Read the model definition and answer for the solid it produces. Units are mm, in the model's axes. A direction names the side the tool comes from. Coordinates: 2 decimals unless noted, no trailing zeros. Write each loop counter-clockwise with the first axis right and the second up, starting at its lowest first coordinate (ties: lowest second). Pieces come first, ordered by that corner, then holes.
(1) Find the intervals of material crossed by probe 1 along Y at (x, z) = (20, 2.4); probe 2 along Y at (x, z) = (0, 3.1); probe 3 along Y at (x, z) = (37, 3.55), in increasing order.
(2) Section D-D on x = 49 is taken. Write down the section's boundary in (y, z), then the cut area to 3 significant figures.
(3) The mould has two halves that part along Y. Classify faces 3 (the cylindrical face through (25.5, 0.07, 2.96)), 4 (the flat face through (30, 0, 6)), 5 (the flat face through (36, -6, 3)): +Y half, -Y half, draft (parallel to the pull), parting line (faces both ways), or undercut.
(4) Given pin 1 (2.5 mm diameter, centred on x = 60, y = 0, fed in from +Z); pin 2 (1.8 mm diameter, centred on x = 24.5, z = 3, fed in from -Y); pin 3 (1.5 mm diameter, centred on y = -2, z = 2, fed in from +X); pin 4 (1 mm diameter, centred on x = 9.5, z = 1, fed in from -Y), each flat-ended and moving along its own axis, determine where each tip first touches the part or whether it passes through.
(5) Section A-A on y = 0 is taken. Write down the section's boundary in (x, z).
(6) Section B-B on x = 20 is taken. Write down the section's boundary in (y, z), then the cut area to 3 significant figures.
(7) Which of the six approach directions +Z, -Z, +X, -X, +Y, -Y give full straight-line access (tool end or side, diameter ignored) to faces 1 (the cylindrical face through (-7.5, -0.16, 2.96)), 2 (the flat face through (35, 6, 3))?
(8) Section C-C on z = 4.9 is taken. Write down the section's boundary in (x, y), then the cut area to 3 significant figures.
from build123d import *

# Parameters (mm, degrees)
EXTRUDE_1_DEPTH    = 6
HOLE_WIZARD_M3_1_D = 3
EXTRUDE_3_DEPTH    = 6


with BuildPart() as part:
    # 草图1 → 凸台-拉伸1 (new body)
    with BuildSketch(Plane.XY):
        with BuildLine():
            Line((0, 6), (60, 6))
            ThreePointArc((60, 6), (66, 0), (60, -6))
            Line((60, -6), (0, -6))
            ThreePointArc((0, -6), (-6, 0), (0, 6))
        make_face()
    extrude(amount=EXTRUDE_1_DEPTH)

    # M3 螺纹孔1 (through all)
    with Locations(Plane.XY.offset(6)):
        with Locations((0, 0), (60, 0), (9, 0), (20, 0), (24, 0)):
            Hole(HOLE_WIZARD_M3_1_D / 2)

    # 草图4 → 凸台-拉伸3 (add)
    with BuildSketch(Plane.XY):
        with BuildLine():
            Line((0, 7.5), (11, 6))
            Line((11, 6), (0, 6))
            ThreePointArc((0, 6), (-6, 0), (0, -6))
            Line((0, -6), (11, -6))
            Line((11, -6), (0, -7.5))
            ThreePointArc((0, -7.5), (-7.5, 0), (0, 7.5))
        make_face()
    extrude(amount=EXTRUDE_3_DEPTH)


solid = part.part
Response:
1. probe 1: y = -6 to -1.5, 1.5 to 6
1. probe 2: y = -7.5 to -1.5, 1.5 to 7.5
1. probe 3: y = -6 to 6
2. outline: (-6, 0) - (6, 0) - (6, 6) - (-6, 6) - close
2. area: 72.0 mm2
3. face 3: undercut
3. face 4: draft
3. face 5: -Y half
4. pin 1: passes through
4. pin 2: stops at y = -6
4. pin 3: stops at x = 65.87
4. pin 4: stops at y = -6.27
5. outline: (-7.5, 0) - (-1.5, 0) - (-1.5, 6) - (-7.5, 6) - close; (1.5, 0) - (7.5, 0) - (7.5, 6) - (1.5, 6) - close; (10.5, 0) - (18.5, 0) - (18.5, 6) - (10.5, 6) - close; (21.5, 0) - (22.5, 0) - (22.5, 6) - (21.5, 6) - close; (25.5, 0) - (58.5, 0) - (58.5, 6) - (25.5, 6) - close; (61.5, 0) - (66, 0) - (66, 6) - (61.5, 6) - close
6. outline: (-6, 0) - (-1.5, 0) - (-1.5, 6) - (-6, 6) - close; (1.5, 0) - (6, 0) - (6, 6) - (1.5, 6) - close
6. area: 54.0 mm2
7. face 1: +Z, -Z, -X
7. face 2: +Z, -Z, +X, +Y
8. outline: (0, -7.5) - (11, -6) - (60, -6) arc R6 ccw to (60, 6) - (11, 6) - (0, 7.5) arc R7.5 ccw to start; hole circle Ø3 at (0, 0); hole circle Ø3 at (9, 0); hole circle Ø3 at (20, 0); hole circle Ø3 at (24, 0); hole circle Ø3 at (60, 0)
8. area: 846 mm2
